Can you work these out from the model? Positions are in its coordinate system, mm. Face numbers are marked on the shaded views. A direction names the side the tool comes from. Give positions to 0.01 mm unless a question says otherwise; leave off trailing zeros. Write each loop counter-clockwise with the first axis right and the second up, starting at its lowest first coordinate (ties: lowest second). Pieces come first, ordered by that corner, then holes. Notation, with made-up numbers: M 32,-18.5 L 79,-18.5 A11 ccw 79,2.5 Z; hole C 89.5,34.25 d5. An arc over 180 degrees is marked long. Write each question's results on one line, items separated by ' | '.
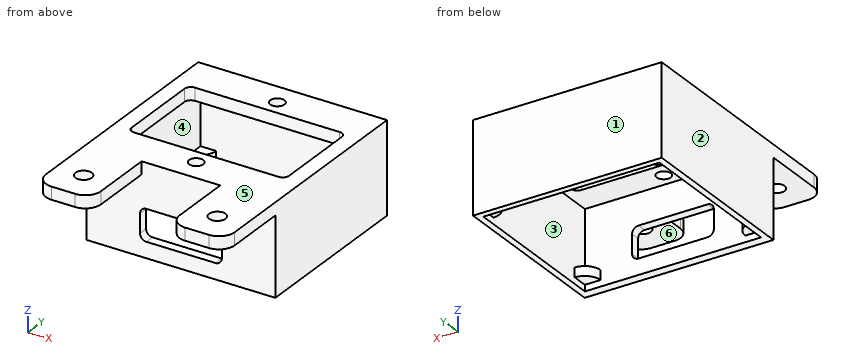
from build123d import *

# Parameters (mm, degrees)
F0_R     = 2.25
F0_R_2   = 2.625
F1_DEPTH = 4
F2_W     = 60
F2_H     = 55
F2_W_2   = 56
F2_H_2   = 50
F3_DEPTH = 25
F5_DEPTH = 25
F6_W     = 5
F6_H     = 5
F7_DEPTH = 5
F8_W     = 56
F8_H     = 50
F9_DEPTH = 2
F10_R    = 4.99999


# Not quite as in the source:
# - a fillet or chamfer is up to 0.001 mm smaller than in the source, because OpenCascade refuses the exact size


with BuildPart() as f1:
    # F0 (on Top) → F1 (new body)
    with BuildSketch(Plane.XY):
        Polygon((30, 27.5), (-30, 27.5), (-30, -27.5), (-12.5000044162, -27.5), (12.5, -27.5), (30, -27.5), align=None)
        with Locations((0, -20)):
            Circle(F0_R, mode=Mode.SUBTRACT)
        with BuildLine():
            ThreePointArc((-25, 13), (-24.4142135624, 14.4142135624), (-23, 15))
            Line((-23, 15), (23, 15))
            ThreePointArc((23, 15), (24.4142135624, 14.4142135624), (25, 13))
            Line((25, 13), (25, -13))
            ThreePointArc((25, -13), (24.4142135624, -14.4142135624), (23, -15))
            Line((23, -15), (-23, -15))
            ThreePointArc((-23, -15), (-24.4142135624, -14.4142135624), (-25, -13))
            Line((-25, -13), (-25, 13))
        make_face(mode=Mode.SUBTRACT)
        with Locations((0, 20)):
            Circle(F0_R, mode=Mode.SUBTRACT)
        with BuildLine():
            Line((-12.5000044162, -27.5), (-30, -27.5))
            Line((-30, -27.5), (-30, -47.5))
            ThreePointArc((-30, -47.5), (-28.5355339059, -51.0355339059), (-25, -52.5))
            Line((-25, -52.5), (-17.5, -52.5))
            ThreePointArc((-17.5, -52.5), (-13.9621173589, -51.0331836094), (-12.5000044162, -47.4933545672))
            Line((-12.5000044162, -47.4933545672), (-12.5000044162, -27.5))
        make_face()
        with Locations((-21.25, -42.5)):
            Circle(F0_R_2, mode=Mode.SUBTRACT)
        with BuildLine():
            Line((30, -47.5), (30, -27.5))
            Line((30, -27.5), (12.5, -27.5))
            Line((12.5, -27.5), (12.5, -47.5))
            ThreePointArc((12.5, -47.5), (13.9644660941, -51.0355339059), (17.5, -52.5))
            Line((17.5, -52.5), (25, -52.5))
            ThreePointArc((25, -52.5), (28.5355339059, -51.0355339059), (30, -47.5))
        make_face()
        with Locations((21.25, -42.5)):
            Circle(F0_R_2, mode=Mode.SUBTRACT)
    extrude(amount=F1_DEPTH)

    # F2 (on face) → F3 (join)
    with BuildSketch(Plane(origin=(0, 0, 0), x_dir=(1, 0, 0), z_dir=(0, 0, -1))):
        Rectangle(F2_W, F2_H)
        with Locations((0, -0.5)):
            Rectangle(F2_W_2, F2_H_2, mode=Mode.SUBTRACT)
    extrude(amount=F3_DEPTH)

    # F4 (on face) → F5 (cut)
    with BuildSketch(Plane(origin=(0, -24.5, 0), x_dir=(-1, 0, 0), z_dir=(0, 1, 0))):
        with BuildLine():
            Line((11, -10), (-11, -10))
            ThreePointArc((-11, -10), (-12.4142135624, -10.5857864376), (-13, -12))
            Line((-13, -12), (-13, -18))
            ThreePointArc((-13, -18), (-12.4142135624, -19.4142135624), (-11, -20))
            Line((-11, -20), (11, -20))
            ThreePointArc((11, -20), (12.4142135624, -19.4142135624), (13, -18))
            Line((13, -18), (13, -12))
            ThreePointArc((13, -12), (12.4142135624, -10.5857864376), (11, -10))
        make_face()
    extrude(amount=-F5_DEPTH, mode=Mode.SUBTRACT)

    # F6 (on face) → F7 (join)
    with BuildSketch(Plane(origin=(0, 0, -25), x_dir=(1, 0, 0), z_dir=(0, 0, -1))):
        with Locations((-25.5, 22)):
            Rectangle(F6_W, F6_H)
        with Locations((25.5, 22)):
            Rectangle(F6_W, F6_H)
        with Locations((25.5, -23)):
            Rectangle(F6_W, F6_H)
        with Locations((-25.5, -23)):
            Rectangle(F6_W, F6_H)
    extrude(amount=-F7_DEPTH)

    # F8 (on face) → F9 (cut)
    with BuildSketch(Plane(origin=(0, 0, -25), x_dir=(1, 0, 0), z_dir=(0, 0, -1))):
        with Locations((0, -0.5)):
            Rectangle(F8_W, F8_H)
    extrude(amount=-F9_DEPTH, mode=Mode.SUBTRACT)

    # F10 (radius 5 in the source; OpenCascade refuses exactly that, so slightly less here)
    f10_edges = [f1.edges().sort_by_distance(p)[0] for p in [
        (-23, -19.5, -21.5),
        (23, -19.5, -21.5),
        (23, 20.5, -21.5),
        (-23, 20.5, -21.5),
    ]]
    fillet(f10_edges, radius=F10_R)


solid = f1.part
Item 1: If I drill on line 1 (Y direction, x = 0, z = 1.9); line 2 (Y direction, x = 21.25, z = 1.05) (3 decimals); line 3 (X direction, y = -13.5, z = -18.25), over which ranges is the centre line in solid material (lowest first)? Write a range as from..to.
Geometry says:
line 1: y = -27.5..-22.25, -17.75..-15, 15..17.75, 22.25..27.5 | line 2: y = -52.5..-45.125, -39.875..-15, 15..27.5 | line 3: x = -30..-28, 28..30
Item 2: I want a section at C-C, the plane z = -3. Please give me the cut outline in (x, y), and give its area (3 significant figures).
Geometry says:
outline: M -30,-27.5 L 30,-27.5 L 30,27.5 L -30,27.5 Z; hole M -28,-24.5 L 28,-24.5 L 28,25.5 L -28,25.5 Z | area: 500 mm2
Item 3: I want a section at B-B, the plane x = -4. Please give me the cut outline in (y, z), and give its area (3 significant figures).
Geometry says:
outline: M -27.5,-25 L -24.5,-25 L -24.5,-20 L -27.5,-20 Z; M -27.5,-10 L -24.5,-10 L -24.5,0 L -15,0 L -15,4 L -27.5,4 Z; M 15,0 L 25.5,0 L 25.5,-25 L 27.5,-25 L 27.5,4 L 15,4 Z | area: 195 mm2
Item 4: Thinking about a two-plate mould opening in X: for the marked faces 1, 2 and 3, which applies, +X half, -X half, draft (parallel to the pull), parting line (faces both ways), or undercut?
Geometry says:
face 1: draft | face 2: -X half | face 3: undercut
Item 5: I'm going to push flat-ended pins straight in: pin 1 (4 mm diameter, centred on x = 15.5, z = -18, fed in from -Y); pin 2 (9 mm diameter, centred on x = 21, y = -44, fed in from -Z). Where does each tip first touch, or does it pass through?
Geometry says:
pin 1: stops at y = -27.5 | pin 2: stops at z = 0
Item 6: For the marked faces 4, 5 and 6, which set-ups out of +Z, -Z, +X, -X, +Y, -Y let a thin tool reach every point of the face, with its end or its side?
Geometry says:
face 4: none | face 5: +Z, +X, -X, +Y, -Y | face 6: -Z, +X, -X, -Y
Item 7: I want a section at A-A, the plane y = -42.5. Please give me the cut outline in (x, z) (3 decimals).
Geometry says:
outline: M -30,0 L -23.875,0 L -23.875,4 L -30,4 Z; M -18.625,0 L -12.5,0 L -12.5,4 L -18.625,4 Z; M 12.5,0 L 18.625,0 L 18.625,4 L 12.5,4 Z; M 23.875,0 L 30,0 L 30,4 L 23.875,4 Z
Item 8: I want a section at D-D, the plane z = -16.25. Please give me the cut outline in (x, y), and give its area (3 significant figures).
Geometry says:
outline: M -30,-27.5 L -13,-27.5 L -13,-24.5 L -28,-24.5 L -28,25.5 L 28,25.5 L 28,-24.5 L 13,-24.5 L 13,-27.5 L 30,-27.5 L 30,27.5 L -30,27.5 Z | area: 422 mm2
